Could you check a few things on this model? Use its own coordinates, in mm. A direction names the side the tool comes from. Round coordinates to 2 decimals unless told otherwise and drop trailing zeros. Loops run counter-clockwise (first coordinate to the right, second up) from the corner with the lowest first, then second, coordinate; pieces in that order, holes last. Notation, with made-up numbers: (-1, 34) -> (23, 34) arc R17 cw to (23, 47) -> close; hole circle Ø6 at (21.25, 64). An arc over 180 degrees is marked (long way). One line per item, written item: value.
```python
from build123d import *

# Parameters (mm, degrees)
BOSS_EXTRU_1_DEPTH = 2
BOSS_EXTRU_2_DEPTH = 1


with BuildPart() as part:
    # Esquisse1 → Boss.-Extru.1 (new body)
    with BuildSketch(Plane.XY):
        with BuildLine():
            Line((-13.186835109, -48.813164891), (-1.838477631, -60.161522369))
            ThreePointArc((-1.838477631, -60.161522369), (0, -59.4), (1.838477631, -60.161522369))
            Line((1.838477631, -60.161522369), (13.443252333, -48.599927693))
            Line((13.443252333, -48.599927693), (13.526323228, -3.099888238))
            ThreePointArc((13.526323228, -3.099888238), (10.400079466, 0.022196444), (13.570710678, 3.099193443))
            Line((13.570710678, 3.099193443), (13.570710678, 48.429289322))
            Line((13.570710678, 48.429289322), (1.838477631, 60.161522369))
            ThreePointArc((1.838477631, 60.161522369), (0, 59.4), (-1.838477631, 60.161522369))
            Line((-1.838477631, 60.161522369), (-13.103328579, 48.983053521))
            Line((-13.103328579, 48.983053521), (-13.103328579, 3.074516512))
            ThreePointArc((-13.103328579, 3.074516512), (-10.4, 0), (-13.103328579, -3.074516512))
            Line((-13.103328579, -3.074516512), (-13.186835109, -48.813164891))
        make_face()
    extrude(amount=BOSS_EXTRU_1_DEPTH)

    # Esquisse2 → Boss.-Extru.2 (add)
    with BuildSketch(Plane.XY.offset(2)):
        Polygon((0, 65.151280821), (-15.028155385, 50.123125436), (-15.028155385, -50.75260641), (0, -65.780761795), (14.971844615, -50.80891718), (14.971844615, 50.179436206), align=None)
    extrude(amount=BOSS_EXTRU_2_DEPTH)


solid = part.part
```
Item 1: I need wall thicknesses on line 1 (X direction, y = 10.5, z = 0.8); line 2 (Y direction, x = -12.5, z = 0.7); line 3 (X direction, y = -6, z = 0.8). Which ranges of each line are inside material? Lowest first, please. Write a range as from..to.
Output:
line 1: x = -13.1..13.57
line 2: y = -49.5..-2.93, 2.93..49.58
line 3: x = -13.11..13.52
Item 2: If we section it at A-A on z = 1.05: List the corners of the cut face in (x, y) for me.
Output:
outline: (-13.19, -48.81) -> (-1.84, -60.16) arc R2.6 cw to (1.84, -60.16) -> (13.44, -48.6) -> (13.53, -3.1) arc R3.1 cw (long way) to (13.57, 3.1) -> (13.57, 48.43) -> (1.84, 60.16) arc R2.6 cw to (-1.84, 60.16) -> (-13.1, 48.98) -> (-13.1, 3.07) arc R3.1 cw to (-13.1, -3.07) -> close
Item 3: For faces 1 (the face through (-7.62, -58.16, 2.49)), 2 (the face through (0, 1, 0)), 3 (the face through (7.56, -54.46, 0.99)), 4 (the face through (8, 54, 1)), 5 (the face through (-7.39, 54.65, 0.99)), which set-ups out of +Z, -Z, +X, -X, +Y, -Y let a thin tool reach every point of the face, with its end or its side?
Output:
face 1: +Z, -Z, -X, -Y
face 2: -Z, +X, -X, +Y, -Y
face 3: -Z, +X, -Y
face 4: -Z, +X, +Y
face 5: -Z, -X, +Y
Item 4: If we section it at B-B on y = 0: List the corners of the cut face in (x, z) for me, plus the area to 3 significant figures.
Output:
outline: (-15.03, 2) -> (-10.4, 2) -> (-10.4, 0) -> (10.4, 0) -> (10.4, 2) -> (14.97, 2) -> (14.97, 3) -> (-15.03, 3) -> close
area: 71.6 mm²
Item 5: Will these pins go through, and if not, where does the flat tip stop? pin 1 Ø1.6 at (y, z) = (17, 1) entering from -X; pin 2 Ø1.5 at (x, z) = (-10.5, 2) entering from +Y.
Output:
pin 1: stops at x = -13.1
pin 2: stops at y = 55.4
Item 6: If we mould it in two halves opening along Y, with no side actions, what happens to faces 6 (the face through (-7.41, 57.74, 2.49)), 7 (the face through (-8, -54, 1)), 8 (the face through (-10.4, 0.1, 1))? For each: released by +Y, released by -Y, zero draft, split by the parting line, or undercut.
Output:
face 6: released by +Y
face 7: released by -Y
face 8: undercut
Item 7: If we section it at C-C on x = -11.75: List the corners of the cut face in (y, z) for me, plus the area to 3 significant figures.
Output:
outline: (-54.03, 2) -> (-50.25, 2) -> (-50.25, 0) -> (-2.56, 0) -> (-2.56, 2) -> (2.56, 2) -> (2.56, 0) -> (50.33, 0) -> (50.33, 2) -> (53.4, 2) -> (53.4, 3) -> (-54.03, 3) -> close
area: 298 mm²
